```python
from build123d import *

# Parameters (mm, degrees)
F0_R          = 27.5
F1_DEPTH      = 150
F3_DEPTH      = 27.5
F3_DEPTH_BACK = 27.5


with BuildPart() as f1:
    # F0 (on Top) → F1 (new body)
    with BuildSketch(Plane.XY):
        Circle(F0_R)
    extrude(amount=F1_DEPTH)


with BuildPart() as f3:
    # F2 (on Front) → F3 (new body, two sides)
    with BuildSketch(Plane.XZ) as f3_sk:
        Polygon((27.5, 153), (-29.5, 153), (27.5, 98), align=None)
    extrude(amount=F3_DEPTH)
    extrude(f3_sk.sketch, amount=-F3_DEPTH_BACK)


with BuildPart() as f1_1:
    add(f1.part)

    # F4: cut F3
    add(f3.part, mode=Mode.SUBTRACT)


solid = f1_1.part
```
Read the model definition and answer for the solid it produces. Units are mm, in the model's axes. Coordinates: 2 decimals unless noted, no trailing zeros. Write each loop counter-clockwise with the first axis right and the second up, starting at its lowest first coordinate (ties: lowest second). Pieces come first, ordered by that corner, then holes. Notation, with made-up numbers: (-14.75, 49.5) - (37.25, 49.5) arc R36 ccw to (37.25, 84.5) - close; hole circle Ø1 at (72, 5.25). An arc over 180 degrees is marked (long way). Answer as a JSON object with one key per item and string values. Group by question number.
1. A cutting plane is placed at A-A (y = 0). Determine the outline of the cut face in (x, z), plus the area to 3 significant figures.
2. Consider L1, parallel to Y at x = -1, z = 51; L2, parallel to Z at x = -14.5, y = -3.5; L3, parallel to X at y = 12, z = 8.5. Determine where each line is inside the solid, lowest interval first. Write a range as [from, to].
3. A cutting plane is placed at B-B (z = 84). Determine the outline of the cut face in (x, y).
4. A cutting plane is placed at D-D (y = -12.5). Determine the outline of the cut face in (x, z), plus the area to 3 significant figures.
5. A cutting plane is placed at C-C (x = 0). Determine the outline of the cut face in (y, z).
6. Each of these flat-tipped pins is pushed along its axis until it touches: P1, Ø1.5, axis at x = 9.5, z = 54, coming from the -Y side; P2, Ø6, axis at y = -18, z = 117, coming from the -X side; P3, Ø2, axis at x = -8, y = -15.5, coming from the +Z side. Where does it stop, or does it pass through?
Worked out:
{
 "1": {"outline": "(-27.5, 0) - (27.5, 0) - (27.5, 98) - (-26.39, 150) - (-27.5, 150) - close", "area": "6,850 mm²"},
 "2": {"L1": "y = [-27.48, 27.48]", "L2": "z = [0, 138.53]", "L3": "x = [-24.74, 24.74]"},
 "3": {"outline": "circle Ø55 at (0, 0)"},
 "4": {"outline": "(-24.49, 0) - (24.49, 0) - (24.49, 100.9) - (-24.49, 148.17) - close", "area": "6,100 mm²"},
 "5": {"outline": "(-27.5, 0) - (27.5, 0) - (27.5, 124.54) - (-27.5, 124.54) - close"},
 "6": {"P1": "stops at y = -26.07", "P2": "stops at x = -23.05", "P3": "stops at z = 133.22"}
}
